Design review of the part built by this model. Coordinates are the model's own, in mm. A direction names the side the tool comes from. Coordinates: 2 decimals unless noted, no trailing zeros. Write each loop counter-clockwise with the first axis right and the second up, starting at its lowest first coordinate (ties: lowest second). Pieces come first, ordered by that corner, then holes. Notation, with made-up numbers: (-40, 45) - (-30, 45) arc R18 cw to (-30, 77) - close; hole circle Ø9 at (27.5, 58). An arc over 180 degrees is marked (long way). Answer as CSV lines item,"result". Start each with the question number.
Q1. We need section D-D (z = 18). Write out the cut boundary in (x, y).
Q2. We need section B-B (z = -2.5). Write out the cut boundary in (x, y).
Q3. Clearance check with flat-ended pins moving along their axes: pin 1 (1 mm diameter, centred on x = -6, z = -6, fed in from -Y); pin 2 (12 mm diameter, centred on x = 7.5, y = 9, fed in from +Z); pin 3 (2 mm diameter, centred on y = 7, z = 2.5, fed in from -X); pin 4 (1 mm diameter, centred on x = 2.5, z = 1.5, fed in from +Y). State where each tip first meets the part, or that it passes through.
Q4. For line 1 along Y through (x, z) = (7.5, -4); line 2 along Z through (x, y) = (-5.25, 11); line 3 along Y through (x, z) = (-8.25, -18), list the stretches that pass through material, from the lowest coordinate up. Write a range as [from, to].
Q5. Machinability: for faces 1 (the face through (10, -6, 0)), 2 (the face through (-10.2, 3.3, -35.9)), which of the approach directions +Z, -Z, +X, -X, +Y, -Y give a long, thin tool a straight path to every point of the face, cutting with its end or side? Answer none if there is none.
Autodesk Inventor part; units mm, degrees
ref_plane "YZ Plane" through (0, 0, 0) normal (1, 0, 0) x (0, 1, 0)
ref_plane "XZ Plane" through (0, 0, 0) normal (0, 1, 0) x (-1, 0, 0)
ref_plane "XY Plane" through (0, 0, 0) normal (0, 0, 1) x (1, 0, 0)
sketch "Sketch1" plane through (0, 0, 0) normal (0, 0, 1) x (1, 0, 0)
  line L0 (-8.128, 7.8935) -> (8.128, 7.8935)
  line L1 (-8.0668, -7.9561) -> (8.0668, -7.9561)
  arc A0 (-8.128, 7.8935) -> (-8.0668, -7.9561) centre (0, 0) ccw
  arc A1 (8.0668, -7.9561) -> (8.128, 7.8935) centre (0, 0) ccw
  line L2 (0, 7.8935) -> (0, -7.9561)
  dimension "d8" = 15.8496
  dimension "d9" = 16.256
extrude "Extrusion1" add sketch "Sketch1" along normal blind 26.4922
sketch "Sketch2" plane through (0, 0, 0) normal (0, 0, -1) x (-0.0038611, 0.9999925, 0)
  line L0 (-7.956, -11.1178) -> (14.2944, -11.1178)
  line L1 (14.2944, -11.1178) -> (14.2944, 11.0564)
  line L2 (14.2944, 11.0564) -> (-7.956, 11.0564)
  line L3 (-7.956, 11.0564) -> (-7.956, -11.1178)
  line L4 (-4.7868, -0.0614) -> (-7.956, -0.0307)
  point P0 (0, 0)
  dimension "d3" = 22.2504
  dimension "d4" = 22.1742
extrude "Extrusion2" add sketch "Sketch2" along normal blind 36.83
fillet "Fillet1" radius 3.175 2 edges at (-11.13, 3.1262, -36.83) (11.0441, 3.2119, -36.83)
sketch "Sketch4" plane through (0, 0, 26.4922) normal (0, 0, 1) x (0.0038611, -0.9999925, 0)
  point P0 (0, 0)
  point P1 (-14.2944, -11.1178)
sketch "Sketch6" plane through (11.087, -7.9133, -33.655) normal (0.0038611, -0.9999925, 0) x (0.9999925, 0.0038611, 0)
  line L0 (-13.3136, 11.6068) -> (-8.7992, 11.6068)
  line L1 (-13.8088, 7.0188) -> (-8.3039, 7.0188)
  arc A0 (-13.3136, 11.6068) -> (-13.8088, 7.0188) centre (-11.0564, 9.0424) ccw
  arc A1 (-8.3039, 7.0188) -> (-8.7992, 11.6068) centre (-11.0564, 9.0424) ccw
  point P0 (-11.0564, 33.655)
extrude "Extrusion3" add sketch "Sketch6" along normal blind 5.207
properties part number "cwmotor"
Results list:
1,outline,"(-8.13, 7.89) arc R11.33 ccw to (-8.07, -7.96) - (8.07, -7.96) arc R11.33 ccw to (8.13, 7.89) - close"
2,outline,"(-11.17, 14.25) - (-11.09, -8) - (11.09, -7.91) - (11, 14.34) - close"
3,pin 1,"stops at y = -7.98"
3,pin 2,"stops at z = 26.49"
3,pin 3,"stops at x = -9.61"
3,pin 4,"stops at y = 7.89"
4,line 1,"y = [-7.93, 14.32]"
4,line 2,"z = [-36.83, 0]"
4,line 3,"y = [-7.99, 14.26]"
5,face 1,"+Z, +X, -Y"
5,face 2,"-Z, -X, -Y"
